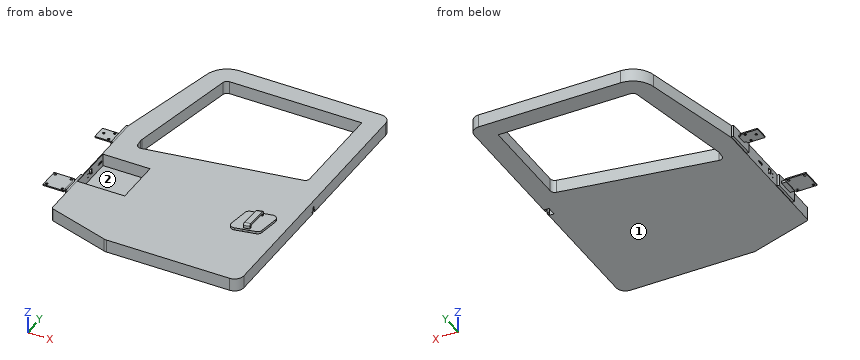
from build123d import *

# Parameters (mm, degrees)
BOSS_EXTRUDE1_DEPTH     = 34.925
BOSS_EXTRUDE2_DEPTH     = 12.7
BOSS_EXTRUDE4_DEPTH     = 38.1
CUT_EXTRUDE6_DEPTH      = 1209.353123139
CUT_EXTRUDE6_DEPTH_BACK = 1209.353123139
SKETCH6_W               = 15.24
SKETCH6_H               = 112.550701787
FILLET5_R               = 10.16
SKETCH7_W               = 63.5
SKETCH7_H               = 152.4
BOSS_EXTRUDE5_DEPTH     = 12.7
SKETCH16_W              = 254
SKETCH16_H              = 254
CUT_EXTRUDE8_DEPTH      = 66.675
SKETCH20_R              = 2.54
SKETCH20_W              = 12.7
SKETCH20_H              = 25.4
CUT_EXTRUDE12_DEPTH     = 3.81
SKETCH21_R              = 6.35
SKETCH21_W              = 12.7
SKETCH21_H              = 53.975
BOSS_EXTRUDE8_DEPTH     = 3.175
SKETCH26_W              = 25.4
SKETCH26_H              = 85.725
BOSS_EXTRUDE12_DEPTH    = 6.35
SKETCH27_W              = 112.7125
SKETCH27_H              = 111.125
SKETCH27_R              = 6.35
BOSS_EXTRUDE13_DEPTH    = 3.175
SKETCH28_R              = 3
CUT_EXTRUDE13_DEPTH     = 3.81
CUT_EXTRUDE14_DEPTH     = 2.54
CUT_EXTRUDE15_DEPTH     = 38.1
SKETCH31_R              = 2.54
CUT_EXTRUDE16_DEPTH     = 10.668


with BuildPart() as part:
    # Sketch2 → Boss-Extrude1 (new, symmetric)
    with BuildSketch(Plane.XY):
        with BuildLine():
            Line((-524.472141427, -657.200845349), (-194.857891611, -759.729501192))
            ThreePointArc((-194.857891611, -759.729501192), (-187.400192227, -761.445624463), (-179.769325902, -762.022025636))
            Line((-179.769325902, -762.022025636), (482.6, -762.022025636))
            ThreePointArc((482.6, -762.022025636), (518.521024484, -747.14305012), (533.4, -711.222025636))
            Line((533.4, -711.222025636), (533.4, 711.177974364))
            ThreePointArc((533.4, 711.177974364), (518.521024484, 747.098998848), (482.6, 761.977974364))
            Line((482.6, 761.977974364), (-281.22987981, 761.977974364))
            ThreePointArc((-281.22987981, 761.977974364), (-361.995192132, 732.98799592), (-405.888305034, 659.253003111))
            Line((-405.888305034, 659.253003111), (-533.4, 116.92602354))
            Line((-533.4, 116.92602354), (-533.4, -645.07397646))
            ThreePointArc((-533.4, -645.07397646), (-530.927321158, -652.603378956), (-524.472141427, -657.200845349))
        make_face()
        with BuildLine():
            Line((-306.172257077, 639.777746889), (-423.021910153, 45.403882754))
            ThreePointArc((-423.021910153, 45.403882754), (-423.905333497, 38.283472292), (-423.776767691, 31.109620274))
            Line((-423.776767691, 31.109620274), (-421.145810725, 1.492076496))
            ThreePointArc((-421.145810725, 1.492076496), (-411.377161007, -16.358363988), (-391.64022517, -21.309940154))
            Line((-391.64022517, -21.309940154), (410.604770812, 113.367925382))
            ThreePointArc((410.604770812, 113.367925382), (425.789915663, 122.010874728), (431.799559386, 138.417378922))
            Line((431.799559386, 138.417378922), (431.8, 660.377974364))
            Line((431.8, 660.377974364), (-281.22987981, 660.377974364))
            ThreePointArc((-281.22987981, 660.377974364), (-297.404640672, 654.562077894), (-306.172257077, 639.777746889))
        make_face(mode=Mode.SUBTRACT)
    extrude(amount=BOSS_EXTRUDE1_DEPTH, both=True)

    # Sketch3 → Boss-Extrude2 (add)
    with BuildSketch(Plane.XY.offset(34.925)):
        with BuildLine():
            Line((360.266650549, -236.97953971), (320.195939672, -245.101046406))
            ThreePointArc((320.195939672, -245.101046406), (306.776022753, -252.553855048), (300.10041124, -266.376833661))
            Line((300.10041124, -266.376833661), (284.73360266, -373.157176687))
            ThreePointArc((284.73360266, -373.157176687), (292.433567965, -395.240613926), (314.920066898, -401.669068776))
            Line((314.920066898, -401.669068776), (354.990777775, -393.547562081))
            Line((354.990777775, -393.547562081), (360.266650549, -236.97953971))
        make_face()
        with BuildLine():
            Line((425.926544142, -223.671633417), (385.855833265, -231.793140113))
            Line((385.855833265, -231.793140113), (380.579960491, -388.361162483))
            Line((380.579960491, -388.361162483), (420.650671368, -380.239655788))
            ThreePointArc((420.650671368, -380.239655788), (434.070588287, -372.786847145), (440.7461998, -358.963868533))
            Line((440.7461998, -358.963868533), (456.11300838, -252.183525507))
            ThreePointArc((456.11300838, -252.183525507), (448.413043075, -230.100088267), (425.926544142, -223.671633417))
        make_face()
        Polygon((385.855833265, -231.793140113), (360.266650549, -236.97953971), (354.990777775, -393.547562081), (380.579960491, -388.361162483), align=None)
    extrude(amount=BOSS_EXTRUDE2_DEPTH)

    # Sketch5 → Boss-Extrude4 (add)
    with BuildSketch(Plane.XY.offset(34.925)):
        Polygon((384.717168986, -375.860232263), (353.492653597, -382.188797573), (356.735325181, -249.357669916), (387.95984057, -243.029104606), align=None)
    extrude(amount=BOSS_EXTRUDE4_DEPTH)

    # Sketch6 → Cut-Extrude6 (cut, two sides: drawn at the far end of the back side and taken through both)
    with BuildSketch(Plane(origin=(393.658065015, -9.60997504, 0), x_dir=(0, 0, -1), z_dir=(0.9997021605932607, -0.02440471481427925, 0)).offset(-CUT_EXTRUDE6_DEPTH_BACK)):
        with Locations((-55.245, -299.924022588)):
            Rectangle(SKETCH6_W, SKETCH6_H)
    extrude(amount=CUT_EXTRUDE6_DEPTH + CUT_EXTRUDE6_DEPTH_BACK, mode=Mode.SUBTRACT)

    # Fillet5
    fillet5_edges = [part.edges().sort_by_distance(p)[0] for p in [
        (372.186129895, -252.807063957, 62.865),
        (369.439362115, -365.324243711, 62.865),
        (369.104911291, -379.024514918, 73.025),
        (372.347582875, -246.193387261, 73.025),
    ]]
    fillet(fillet5_edges, radius=FILLET5_R)

    # Sketch7 → Boss-Extrude5 (add)
    with BuildSketch(Plane(origin=(-533.4, 59.373810393, 0), x_dir=(0, 0, 1), z_dir=(1, 0, 0))):
        with Locations((0, 18.647786854)):
            Rectangle(SKETCH7_W, SKETCH7_H)
        with Locations((0, 475.847786854)):
            Rectangle(SKETCH7_W, SKETCH7_H)
    extrude(amount=-BOSS_EXTRUDE5_DEPTH)

    # Sketch16 → Cut-Extrude8 (cut)
    with BuildSketch(Plane.XY.offset(34.925)):
        with Locations((-402.59, -275.309940154)):
            Rectangle(SKETCH16_W, SKETCH16_H)
    extrude(amount=-CUT_EXTRUDE8_DEPTH, mode=Mode.SUBTRACT)

    # Sketch20 → Cut-Extrude12 (cut)
    with BuildSketch(Plane.ZY.offset(533.4)):
        with Locations(Location((0, -158.772025636, 0), (0, 0, 270))):
            Circle(SKETCH20_R)
        with Locations((0, -193.697025636)):
            Circle(SKETCH20_R)
        with Locations((0, -176.234525636)):
            Rectangle(SKETCH20_W, SKETCH20_H)
    extrude(amount=-CUT_EXTRUDE12_DEPTH, mode=Mode.SUBTRACT)

    # Sketch21 → Boss-Extrude8 (add, symmetric)
    # profile 1 of 2: a face of its own
    with BuildSketch(Plane.XY):
        Polygon((-558.8, 12.677974364), (-558.8, 66.652974364), (-558.8, 77.447974364), (-654.05, 77.447974364), (-654.05, 1.247974364), (-558.8, 1.247974364), align=None)
        with Locations((-584.2, 12.677974364)):
            Circle(SKETCH21_R, mode=Mode.SUBTRACT)
        with Locations((-628.65, 44.427974364)):
            Circle(SKETCH21_R, mode=Mode.SUBTRACT)
        with Locations((-581.025, 66.652974364)):
            Circle(SKETCH21_R, mode=Mode.SUBTRACT)
    # profile 2 of 2: a face of its own
    with BuildSketch(Plane.XY):
        with Locations((-552.45, 39.665474364)):
            Rectangle(SKETCH21_W, SKETCH21_H)
    extrude(amount=BOSS_EXTRUDE8_DEPTH, both=True)

    # Sketch26 → Boss-Extrude12 (add, symmetric)
    with BuildSketch(Plane.XY):
        with Locations((-558.8, -406.422025636)):
            Rectangle(SKETCH26_W, SKETCH26_H)
    extrude(amount=BOSS_EXTRUDE12_DEPTH, both=True)

    # Sketch27 → Boss-Extrude13 (add, symmetric)
    with BuildSketch(Plane.XY):
        with Locations((-627.85625, -406.422025636)):
            Rectangle(SKETCH27_W, SKETCH27_H)
        with Locations((-585.7875, -363.559525636)):
            Circle(SKETCH27_R, mode=Mode.SUBTRACT)
        with Locations((-671.5125, -449.284525636)):
            Circle(SKETCH27_R, mode=Mode.SUBTRACT)
        with Locations((-585.7875, -449.284525636)):
            Circle(SKETCH27_R, mode=Mode.SUBTRACT)
        with Locations((-671.5125, -363.559525636)):
            Circle(SKETCH27_R, mode=Mode.SUBTRACT)
    extrude(amount=BOSS_EXTRUDE13_DEPTH, both=True)

    # Sketch28 → Cut-Extrude13 (cut)
    with BuildSketch(Plane.ZY.offset(533.4)):
        with Locations(Location((-7.705, -258.147025636, 0), (0, 0, 270))):
            Circle(SKETCH28_R)
        with Locations(Location((-7.705, -298.147025636, 0), (0, 0, 270))):
            Circle(SKETCH28_R)
        with Locations(Location((12.295, -298.147025636, 0), (0, 0, 270))):
            Circle(SKETCH28_R)
        with BuildLine():
            Line((9.225, -256.897025636), (22.225, -256.897025636))
            Line((22.225, -256.897025636), (22.225, -282.897025636))
            Line((22.225, -282.897025636), (9.225, -282.897025636))
            ThreePointArc((9.225, -282.897025636), (-3.775, -269.897025636), (9.225, -256.897025636))
        make_face()
    extrude(amount=-CUT_EXTRUDE13_DEPTH, mode=Mode.SUBTRACT)

    # Sketch29 → Cut-Extrude14 (cut)
    with BuildSketch(Plane(origin=(533.4, 0, 0), x_dir=(0, 0, -1), z_dir=(1, 0, 0))):
        with BuildLine():
            Line((27.305, -15.897025636), (34.925, -23.517025636))
            Line((34.925, -23.517025636), (34.925, -15.897025636))
            Line((34.925, -15.897025636), (34.925, -0.022025636))
            Line((34.925, -0.022025636), (27.305, -7.642025636))
            Line((27.305, -7.642025636), (1.938532156, -7.642025636))
            ThreePointArc((1.938532156, -7.642025636), (-2.188967844, -11.769525636), (1.938532156, -15.897025636))
            Line((1.938532156, -15.897025636), (27.305, -15.897025636))
        make_face()
    extrude(amount=-CUT_EXTRUDE14_DEPTH, mode=Mode.SUBTRACT)

    # Sketch30 → Cut-Extrude15 (cut)
    with BuildSketch(Plane(origin=(0, 0, -34.925), x_dir=(-1, 0, 0), z_dir=(0, 0, -1))):
        Polygon((-530.86, -11.769525636), (-530.86, 13.630474364), (-505.46, 13.630474364), (-505.46, -37.169525636), (-530.86, -37.169525636), align=None)
    extrude(amount=-CUT_EXTRUDE15_DEPTH, mode=Mode.SUBTRACT)

    # Sketch31 → Cut-Extrude16 (cut)
    with BuildSketch(Plane(origin=(533.4, 0, 0), x_dir=(0, 0, -1), z_dir=(1, 0, 0))):
        with Locations(Location((24.765, 0.930474364, 0), (0, 0, 90))):
            Circle(SKETCH31_R)
        with Locations(Location((24.765, -24.469525636, 0), (0, 0, 90))):
            Circle(SKETCH31_R)
    extrude(amount=-CUT_EXTRUDE16_DEPTH, mode=Mode.SUBTRACT)


solid = part.part
Could you check a few things on this model? Use its own coordinates, in mm. Face numbers are marked on the shaded views. Give positions to 0.01 mm unless a question says otherwise; leave off trailing zeros. Write each loop counter-clockwise with the first axis right and the second up, starting at its lowest first coordinate (ties: lowest second). Pieces come first, ordered by that corner, then holes. Notation, with made-up numbers: (87.5, 22.25) -> (109.5, 22.25) arc R22 ccw to (109.5, 29.25) -> close; hole circle Ø3 at (5.25, 63.5). An arc over 180 degrees is marked (long way). Write each question's results on one line, items separated by ' | '. Start each with the question number.
Q1. We'd pull the mould along X, two halves only. Please class the marked faces 1 and 2: +X half, -X half, draft (parallel to the pull), parting line (faces both ways), or undercut.
Q2. Suppose I cut it at C-C, the plane x = -466. List the corners of the cut face in (y, z) for me (3 decimals).
Q3. Suppose I cut it at A-A, the plane x = 118. List the corners of the cut face in (y, z) for me (3 decimals), and give its area (3 significant figures).
Q4. I need wall thicknesses on probe 1 along X at (y, z) = (-225, 11); probe 2 along Y at (x, z) = (-81.5, 23.5); probe 3 along Y at (x, z) = (-544, 6). Which ranges of each line are inside material? Lowest first, please.
Q5. Suppose I cut it at B-B, the plane y = 343. List the corners of the cut face in (x, z) for me (3 decimals), and give its area (3 significant figures).
Q6. I'm going to push flat-ended pins straight in: pin 1 Ø14 at (x, z) = (-555.5, -0.5) entering from +Y; pin 2 Ø7 at (y, z) = (-258.15, -7.7) entering from -X; pin 3 Ø8 at (x, y) = (-373.5, -493.5) entering from +Z (3 decimals); pin 4 Ø7.5 at (x, y) = (-671.51, -363.56) entering from -Z. Where does each tip first touch, or does it pass through?
Outcome:
1) face 1: draft | face 2: undercut
2) outline: (-675.389, -34.925) -> (403.589, -34.925) -> (403.589, 34.925) -> (-148.31, 34.925) -> (-148.31, -31.75) -> (-402.31, -31.75) -> (-402.31, 34.925) -> (-675.389, 34.925) -> close
3) outline: (-762.022, -34.925) -> (64.247, -34.925) -> (64.247, 34.925) -> (-762.022, 34.925) -> close; (660.378, -34.925) -> (761.978, -34.925) -> (761.978, 34.925) -> (660.378, 34.925) -> close | area: 64,800 mm2
4) probe 1: -533.4 to -529.59, -275.59 to 533.4 | probe 2: -762.02 to 30.76, 660.38 to 761.98 | probe 3: -492.67 to -340.27, -35.47 to 116.93
5) outline: (-480.246, -34.925) -> (-364.517, -34.925) -> (-364.517, 34.925) -> (-480.246, 34.925) -> close; (431.8, -34.925) -> (533.4, -34.925) -> (533.4, 34.925) -> (431.8, 34.925) -> close | area: 15,200 mm2
6) pin 1: y = 77.45 | pin 2: x = -533.4 | pin 3: z = 34.925 | pin 4: through
